Read the model definition and answer for the solid it produces. Units are mm, in the model's axes. Face numbers are marked on the shaded views. Coordinates: 2 decimals unless noted, no trailing zeros. One line per question, with ' | ' between items. Start each with the question number.
```python
from build123d import *

# Parameters (mm, degrees)
BOSS_EXTRUDE1_DEPTH = 1
BOSS_EXTRUDE2_START = -1
BOSS_EXTRUDE2_DEPTH = 8
CUT_EXTRUDE1_DEPTH  = 18
FILLET2_R           = 1
BOSS_EXTRUDE3_START = 8
BOSS_EXTRUDE3_DEPTH = 1


with BuildPart() as part:
    # Sketch1 → Loft2 section 0
    with BuildSketch(Plane(origin=(0, 0, 0), x_dir=(1, 0, 0), z_dir=(0, 1, 0))):
        with BuildLine():
            Line((9, -9), (-9, -9))
            Line((-9, -9), (-9, 9))
            Line((-9, 9), (9, 9))
            Line((9, 9), (9, -9))
        make_face()
    # Sketch3 → Loft2 section 1
    with BuildSketch(Plane(origin=(0, 9, 0), x_dir=(1, 0, 0), z_dir=(0, 1, 0))):
        with BuildLine():
            Line((0, 9), (-7, 9))
            Line((-7, 9), (-7, -5))
            Line((-7, -5), (7, -5))
            Line((7, -5), (7, 9))
            Line((7, 9), (0, 9))
        make_face()
    loft()

    # Cut-Loft3: read off the stored shape, not the designer's step
    # Cut-Loft3: loft between two sections, ruled curve by curve
    cut_loft3_from = [
        Edge.make_line((8, 0, -8), (8, 0, 8)),
        Edge.make_line((-8, 0, -8), (8, 0, -8)),
        Edge.make_line((-8, 0, 8), (-8, 0, -8)),
        Edge.make_line((8, 0, 8), (-8, 0, 8)),
    ]
    cut_loft3_to = [
        Edge.make_line((6, 9, -8), (6, 9, 4)),
        Edge.make_line((-6, 9, -8), (6, 9, -8)),
        Edge.make_line((-6, 9, 4), (-6, 9, -8)),
        Edge.make_line((6, 9, 4), (-6, 9, 4)),
    ]
    cut_loft3 = Solid(Shell([*[Face.make_surface_from_curves(cut_loft3_from[k], cut_loft3_to[k]) for k in range(4)], Face(Wire(cut_loft3_from)), Face(Wire(cut_loft3_to))]))
    add(cut_loft3, mode=Mode.SUBTRACT)

    # Sketch3<8> → Boss-Extrude1 (add)
    with BuildSketch(Plane(origin=(0, 9, 0), x_dir=(1, 0, 0), z_dir=(0, 1, 0))):
        Polygon((0, 9), (-7, 9), (-7, -5), (7, -5), (7, 9), align=None)
    extrude(amount=-BOSS_EXTRUDE1_DEPTH)

    # Sketch9 → Boss-Extrude2 (add)
    with BuildSketch(Plane(origin=(0, 9, 0), x_dir=(1, 0, 0), z_dir=(0, 1, 0)).offset(BOSS_EXTRUDE2_START)):
        with BuildLine():
            ThreePointArc((2.5, 2), (1.767766953, 3.767766953), (0, 4.5))
            Line((0, 4.5), (0, 4))
            ThreePointArc((0, 4), (0.252008585, 3.984059393), (0.5, 3.936491673))
            ThreePointArc((0.5, 3.936491673), (1.414213562, 3.414213562), (1.936491673, 2.5))
            ThreePointArc((1.936491673, 2.5), (1.984059393, 2.252008585), (2, 2))
            ThreePointArc((2, 2), (1.984059393, 1.747991415), (1.936491673, 1.5))
            ThreePointArc((1.936491673, 1.5), (1.414213562, 0.585786438), (0.5, 0.063508327))
            ThreePointArc((0.5, 0.063508327), (0.252008585, 0.015940607), (0, 0))
            Line((0, 0), (0, -0.5))
            ThreePointArc((0, -0.5), (1.767766953, 0.232233047), (2.5, 2))
        make_face()
        with BuildLine():
            Line((0, 4), (0, 4.5))
            ThreePointArc((0, 4.5), (-2.5, 2), (0, -0.5))
            Line((0, -0.5), (0, 0))
            ThreePointArc((0, 0), (-0.252008585, 0.015940607), (-0.5, 0.063508327))
            ThreePointArc((-0.5, 0.063508327), (-1.414213562, 0.585786438), (-1.936491673, 1.5))
            ThreePointArc((-1.936491673, 1.5), (-2, 2), (-1.936491673, 2.5))
            ThreePointArc((-1.936491673, 2.5), (-1.414213562, 3.414213562), (-0.5, 3.936491673))
            ThreePointArc((-0.5, 3.936491673), (-0.252008585, 3.984059393), (0, 4))
        make_face()
        with BuildLine():
            Line((-0.5, 2.5), (-0.5, 3.936491673))
            ThreePointArc((-0.5, 3.936491673), (-1.414213562, 3.414213562), (-1.936491673, 2.5))
            Line((-1.936491673, 2.5), (-0.5, 2.5))
        make_face()
        with BuildLine():
            ThreePointArc((1.936491673, 2.5), (1.414213562, 3.414213562), (0.5, 3.936491673))
            Line((0.5, 3.936491673), (0.5, 2.5))
            Line((0.5, 2.5), (1.936491673, 2.5))
        make_face()
        with BuildLine():
            Line((0.5, 1.5), (0.5, 0.063508327))
            ThreePointArc((0.5, 0.063508327), (1.414213562, 0.585786438), (1.936491673, 1.5))
            Line((1.936491673, 1.5), (0.5, 1.5))
        make_face()
        with BuildLine():
            ThreePointArc((-1.936491673, 1.5), (-1.414213562, 0.585786438), (-0.5, 0.063508327))
            Line((-0.5, 0.063508327), (-0.5, 1.5))
            Line((-0.5, 1.5), (-1.936491673, 1.5))
        make_face()
    extrude(amount=-BOSS_EXTRUDE2_DEPTH)

    # Sketch10 → Cut-Extrude1 (cut)
    with BuildSketch(Plane(origin=(0, 0, -9), x_dir=(-1, 0, 0), z_dir=(0, 0, -1))):
        with BuildLine():
            Line((-7, 9), (7, 9))
            ThreePointArc((7, 9), (0, 8.4960195), (-7, 9))
        make_face()
    extrude(amount=-CUT_EXTRUDE1_DEPTH, mode=Mode.SUBTRACT)

    # Fillet2
    fillet2_edges = [part.edges().sort_by_distance(p)[0] for p in [
        (-8, 4.5, -9),
        (8, 4.5, -9),
        (8, 4.5, 7),
        (-8, 4.5, 7),
    ]]
    fillet(fillet2_edges, radius=FILLET2_R)

    # Sketch12 → Boss-Extrude3 (add)
    with BuildSketch(Plane(origin=(0, 0, 0), x_dir=(1, 0, 0), z_dir=(0, 1, 0)).offset(BOSS_EXTRUDE3_START)):
        with BuildLine():
            Line((3.581786245, 4.240596222), (2.945334125, 4.272419097))
            ThreePointArc((2.945334125, 4.272419097), (1.580068464, 5.534847266), (-0.142959574, 4.835669471))
            ThreePointArc((-0.142959574, 4.835669471), (-0.072742065, 3.461690437), (1.301236968, 3.531907946))
            ThreePointArc((1.301236968, 3.531907946), (1.344877857, 3.934460155), (1.181086076, 4.304764166))
            ThreePointArc((1.181086076, 4.304764166), (1.26486543, 4.372930475), (1.372307239, 4.361890385))
            ThreePointArc((1.372307239, 4.361890385), (1.623671348, 3.567376067), (1.121377086, 2.902441943))
            ThreePointArc((1.121377086, 2.902441943), (-0.231414775, 3.184828144), (-0.539737114, 4.531945481))
            ThreePointArc((-0.539737114, 4.531945481), (-1.819279995, 4.009007276), (-2.205376195, 2.681745404))
            ThreePointArc((-2.205376195, 2.681745404), (-3.016060665, 2.51631725), (-3.646364404, 1.980320066))
            ThreePointArc((-3.646364404, 1.980320066), (-4.327119044, 1.689455161), (-5.014157813, 1.965148837))
            ThreePointArc((-5.014157813, 1.965148837), (-4.281658635, 0.548246446), (-2.76180221, 0.064300293))
            ThreePointArc((-2.76180221, 0.064300293), (-2.037336191, 1.379203145), (-0.787003641, 0.548246446))
            ThreePointArc((-0.787003641, 0.548246446), (-0.886204145, 0.498401478), (-0.957055057, 0.583873164))
            ThreePointArc((-0.957055057, 0.583873164), (-2.00225835, 1.042077327), (-2.507207587, 0.018638396))
            ThreePointArc((-2.507207587, 0.018638396), (-1.297421649, -0.973910564), (0.096724797, -0.26321292))
            ThreePointArc((0.096724797, -0.26321292), (1.566904433, -0.806570536), (2.770449564, 0.197493596))
            ThreePointArc((2.770449564, 0.197493596), (2.019360199, 1.069566472), (2.30803646, 2.183708451))
            ThreePointArc((2.30803646, 2.183708451), (2.838720645, 2.372686483), (3.312040204, 2.067224545))
            ThreePointArc((3.312040204, 2.067224545), (3.292128592, 1.945237225), (3.170141272, 1.965148837))
            ThreePointArc((3.170141272, 1.965148837), (2.944061172, 2.078913386), (2.697636855, 2.021210346))
            ThreePointArc((2.697636855, 2.021210346), (2.333692103, 1.174003789), (2.901024067, 0.447127475))
            ThreePointArc((2.901024067, 0.447127475), (4.865037055, 2.052490742), (3.581786245, 4.240596222))
        make_face()
    extrude(amount=BOSS_EXTRUDE3_DEPTH)


solid = part.part
```
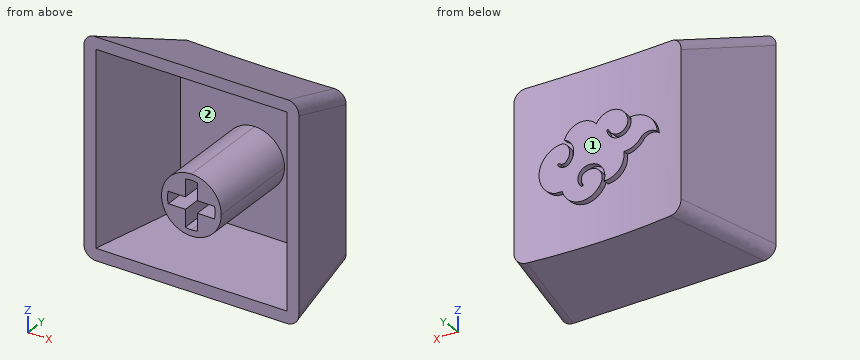
(1) Each of these flat-tipped pins is pushed along its axis until it touches: pin 1 Ø6 at (x, z) = (-2, -4) entering from -Y; pin 2 Ø1.6 at (y, z) = (4, -1) entering from +X; pin 3 Ø1.1 at (x, y) = (-1.5, 6) entering from +Z; pin 4 Ø2 at (y, z) = (3.5, -3) entering from -X. Where does it stop, or does it pass through?
(2) Determine the mould class of the marked faces 1 and 2 for opening direction Z: +Z half, -Z half, draft (parallel to the pull), parting line (faces both ways), or undercut.
(3) Find the intervals of material crossed by probe 1 along X at (y, z) = (4.5, 4.25); probe 2 along Z at (x, y) = (-1.25, 6.75); probe 3 along X at (y, z) = (1.25, -1.75), in increasing order. Write a range as from..to.
(4) Section A-A on y = 5.5 is taken. Give the number of separate pieces and of enclosed holes in the cut face, plus the area to 3 significant figures.
Working result:
1) pin 1: stops at y = 0 | pin 2: stops at x = 8.29 | pin 3: stops at z = 6.58 | pin 4: stops at x = -8.44
2) face 1: draft | face 2: undercut
3) probe 1: x = -8..-7, 7..8 | probe 2: z = -9..-8, -4.17..-2.5, -1.5..0.17, 5..6 | probe 3: x = -8.72..-7.72, -2.49..-1.98, 1.98..2.49, 7.72..8.72
4) separate pieces: 2 | enclosed holes: 2 | area: 70.1 mm2
